Job drawing, mm, ordinate dimensions from the low corner. One solid piece. A direction names the side the tool comes from. Round coordinates to 2 decimals unless told otherwise and drop trailing zeros. Write each loop counter-clockwise with the first axis right and the second up, starting at its lowest first coordinate (ties: lowest second). Pieces come first, ordered by that corner, then holes. Notation, with made-up numbers: M 36,18.5 L 62,18.5 A19 ccw 62,45.5 Z; hole C 50.5,5.25 d9. An arc over 180 degrees is marked long. Answer as a JSON object with one key per item and string values. Group by question number.
1. Drill centre lines: line 1 (Z direction, x = 44.25, y = 19.5); line 2 (Z direction, x = 56.5, y = 125.5); line 3 (Z direction, x = 25.5, y = 118). Where is each one in solid material? Low to high. Write a range as from..to.
2. Band-saw the part on A-A, the plane x = 44.25. Write the cut outline in (y, z).
3. Two-plate mould, pull along Y, no slides. Class the marked faces 1, 2 and 3: +Y half, -Y half, draft (parallel to the pull), parting line (faces both ways), or undercut.
4. Band-saw the part on C-C, the plane z = 9. Write the cut outline in (x, y).
5. Which spindle directions (+Z, -Z, +X, -X, +Y, -Y) get a long thin tool onto all of the face, cutting with end or side? Do the marked faces 4, 5 and 6. Say none if no direction does.
6. Drop flat-ended pins along their axis: pin 1 (5 mm diameter, centred on x = 35, y = 47, fed in from +Z); pin 2 (25 mm diameter, centred on x = 71.5, y = 128, fed in from +Z); pin 3 (5 mm diameter, centred on y = 91, z = 109, fed in from -X). Give the stop position or say it passes through.
7. Band-saw the part on B-B, the plane y = 58. Write the cut outline in (x, z).
8. Band-saw the part on D-D, the plane x = 19. Write the cut outline in (y, z), plus the area to 3 significant figures.
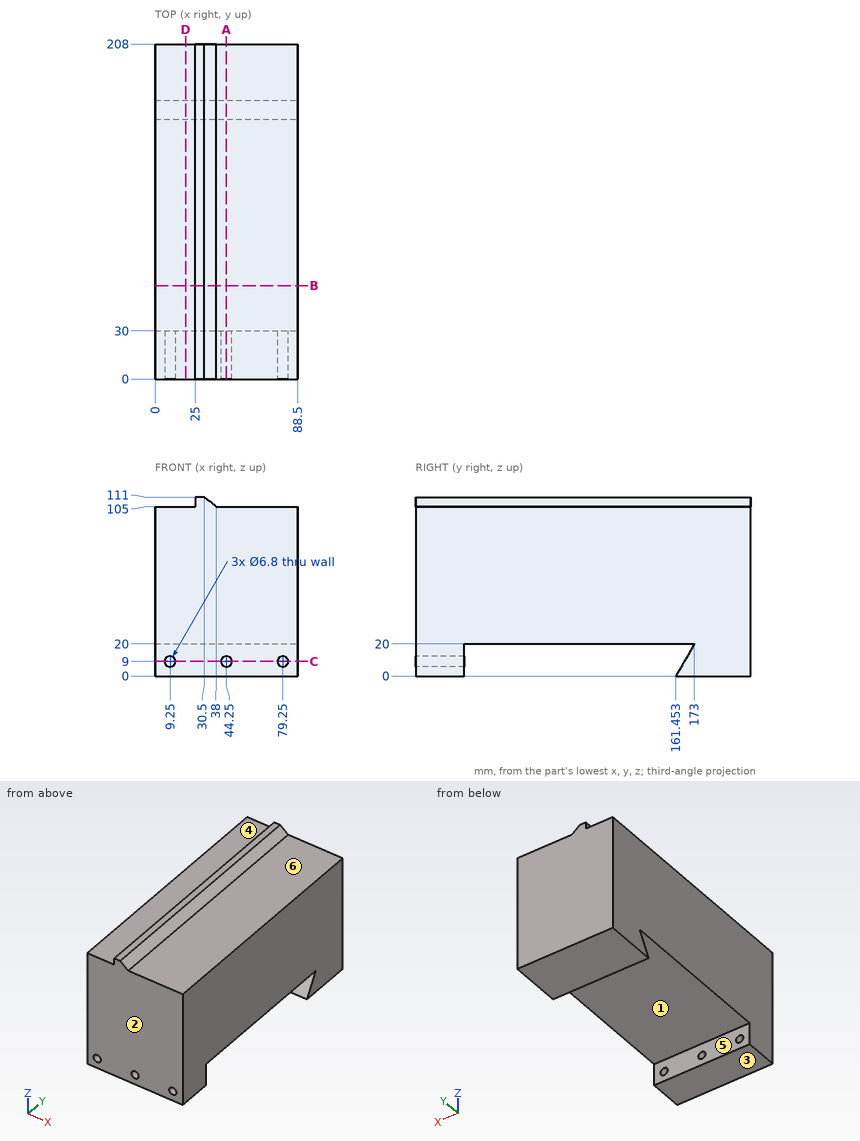
Worked answers:
{
 "1": {"line 1": "z = 0..5.6, 12.4..105", "line 2": "z = 20..105", "line 3": "z = 20..111"},
 "2": {"outline": "M 0,0 L 30,0 L 30,5.6 L 0,5.6 Z; M 0,12.4 L 30,12.4 L 30,20 L 173,20 L 161.45,0 L 208,0 L 208,105 L 0,105 Z"},
 "3": {"face 1": "undercut", "face 2": "-Y half", "face 3": "draft"},
 "4": {"outline": "M 0,0 L 5.85,0 L 5.85,30 L 0,30 Z; M 0,166.65 L 88.5,166.65 L 88.5,208 L 0,208 Z; M 12.65,0 L 40.85,0 L 40.85,30 L 12.65,30 Z; M 47.65,0 L 75.85,0 L 75.85,30 L 47.65,30 Z; M 82.65,0 L 88.5,0 L 88.5,30 L 82.65,30 Z"},
 "5": {"face 4": "+Z, -X, +Y, -Y", "face 5": "-Z, +X, -X", "face 6": "+Z, +X, +Y, -Y"},
 "6": {"pin 1": "stops at z = 109.4", "pin 2": "stops at z = 105", "pin 3": "stops at x = 25"},
 "7": {"outline": "M 0,20 L 88.5,20 L 88.5,105 L 38,105 L 30.5,111 L 25,111 L 25,105 L 0,105 Z"},
 "8": {"outline": "M 0,0 L 30,0 L 30,20 L 173,20 L 161.45,0 L 208,0 L 208,105 L 0,105 Z", "area": "19,100 mm^2"}
}
